from build123d import *

# Parameters (mm, degrees)
EXTRUDE_1_DEPTH     = 190
FILLET_1_R          = 3
FILLET_2_R          = 3
FILLET_3_R          = 3
FILLET_4_R          = 3
SKETCH_2_W          = 263.076218716
SKETCH_2_H          = 173.825805258
CUT_EXTRUDE_1_DEPTH = 1
SKETCH_3_R          = 1.5
EXTRUDE_2_DEPTH     = 5
SKETCH_4_R          = 1.5
EXTRUDE_3_DEPTH     = 5


with BuildPart() as part:
    # 草图1 → 凸台-拉伸1 (new body)
    with BuildSketch(Plane.XY):
        Polygon((-7.851986906, 22.583577614), (-11.052908905, 18.742471216), (204.049049383, -160.50916069), (207.249971381, -156.668054292), align=None)
    extrude(amount=EXTRUDE_1_DEPTH)

    # 圆角1
    fillet_1_edges = [part.edges().sort_by_distance(p)[0] for p in [
        (205.649510382, -158.588607491, 0),
    ]]
    fillet(fillet_1_edges, radius=FILLET_1_R)

    # 圆角2
    fillet_2_edges = [part.edges().sort_by_distance(p)[0] for p in [
        (205.649510382, -158.588607491, 190),
    ]]
    fillet(fillet_2_edges, radius=FILLET_2_R)

    # 圆角3
    fillet_3_edges = [part.edges().sort_by_distance(p)[0] for p in [
        (-9.452447905, 20.663024415, 190),
    ]]
    fillet(fillet_3_edges, radius=FILLET_3_R)

    # 圆角4
    fillet_4_edges = [part.edges().sort_by_distance(p)[0] for p in [
        (-9.452447905, 20.663024415, 0),
    ]]
    fillet(fillet_4_edges, radius=FILLET_4_R)

    # 草图2 → 切除-拉伸1 (cut)
    with BuildSketch(Plane(origin=(7.888650095, 9.466380114, 0), x_dir=(0.76822128, -0.6401844, 0), z_dir=(0.6401844, 0.76822128, 0))):
        with Locations((119.510282494, -95)):
            Rectangle(SKETCH_2_W, SKETCH_2_H)
    extrude(amount=-CUT_EXTRUDE_1_DEPTH, mode=Mode.SUBTRACT)

    # 草图3 → 凸台-拉伸2 (add)
    with BuildSketch(Plane(origin=(0, 0, 0), x_dir=(-1, 0, 0), z_dir=(0, 0, -1))):
        with Locations(Location((-98.098531238, -68.962791538, 0), (0, 0, 180))):  # turned: the seam where the file's is
            Circle(SKETCH_3_R)
    extrude(amount=EXTRUDE_2_DEPTH)

    # 草图4 → 凸台-拉伸3 (add)
    with BuildSketch(Plane.XY.offset(190)):
        with Locations((98.098531238, -68.962791538)):
            Circle(SKETCH_4_R)
    extrude(amount=EXTRUDE_3_DEPTH)


solid = part.part
Geometry check sheet. Reference: the model listing, model coordinates, mm. A direction names the side the tool comes from. Give positions to 0.01 mm unless a question says otherwise; leave off trailing zeros. Order: outer loops, then holes, each group sorted by start corner. A loop starts at its lowest first (then second) coordinate and runs counter-clockwise, first axis right, second up.
1) Cross-section at A-A (z = 82.5). Record the boundary of the cut face in (x, y).
Results are:
outline: (-11.05, 18.74) - (204.05, -160.51) - (207.25, -156.67) - (200.75, -151.25) - (200.11, -152.02) - (-1.99, 16.4) - (-1.35, 17.17) - (-7.85, 22.58) - close
2) Draft check along Z on faces 1 (the flat face through (98, -66, 8.087)), 2 (the cylindrical face through (205.015, -158.014, 0.902)), 3 (the flat face through (106, -75, 190)). Enter one of: released by +Z, released by -Z, zero draft, split by the parting line, or undercut.
Results are:
face 1: undercut
face 2: released by -Z
face 3: released by +Z
3) Tool access check on faces 4 (the flat face through (98, -66, 181.913)), 5 (the cylindrical face through (205.015, -158.014, 189.098)). Record the directions out of +Z, -Z, +X, -X, +Y, -Y that give a thin tool (end or side, any length) a straight path to the whole face; none if there is none.
Results are:
face 4: +X, +Y
face 5: +Z, +X, -Y
4) Cross-section at B-B (y = -73.5). Record the boundary of the cut face in (x, z).
Results are:
outline: (99.64, 0) - (107.45, 0) - (107.45, 8.09) - (105.89, 8.09) - (105.89, 181.91) - (107.45, 181.91) - (107.45, 190) - (99.64, 190) - close
5) Gauge pin test, flat ends, axial feed: pin 1 (5 mm diameter, centred on y = -109.5, z = 105.5, fed in from +X); pin 2 (8 mm diameter, centred on y = -115.5, z = 103.5, fed in from +X); pin 3 (10 mm diameter, centred on x = 25, z = 22.5, fed in from -Y). Record the tip position at first contact, or that the pin passes through.
Results are:
pin 1: stops at x = 152.09
pin 2: stops at x = 161.09
pin 3: stops at y = -15.47
6) Material ranges on probe 1 along Y at (x, z) = (-1.5, 112); probe 2 along X at (y, z) = (-106, 66.5); probe 3 along X at (y, z) = (-99.5, 27), recorded low to high.
Results are:
probe 1: y = 10.78 to 15.99, 16.99 to 17.29
probe 2: x = 138.64 to 144.89
probe 3: x = 130.84 to 137.09
